Input: part model. Units: mm. Frame: model coordinates. Face numbers are marked on the shaded views. A direction names the side the tool comes from. Give positions to 0.01 mm unless a question says otherwise; leave off trailing zeros. One line per item, written item: value. Start each with the question number.
(1) Access query for the marked faces 1, 2 and 3. Directions: +Z, -Z, +X, -X, +Y, -Y. A direction counts if a zero-diameter tool reaches every point of the face in a straight line with its end or side. Return the directions, or none.
(2) Pull-direction query (X, two-part tool) for the marked faces 4, 5, 6 and 7; classes: released by +X, released by -X, zero draft, split by the parting line, or undercut.
(3) Ray query, line 1 along Z through (x, y) = (0, -22); line 2 along Y through (x, z) = (0, 8) (3 decimals); line 3 along Z through (x, y) = (0, 20.7). Return the intervals inside material, ascending. Write a range as from..to.
(4) Pin query (flat end, axial travel): P1, Ø1.5, axis at y = -1, z = -5, coming from the +X side; P2, Ø6, axis at y = 12.5, z = -14.5, coming from the -X side; P3, Ø6, axis at x = 18.5, z = 10, coming from the +Y side. Return the tip coordinate at first contact, or that it passes through.
```python
from build123d import *

# Parameters (mm, degrees)
SKETCH_2_W                       = 64.02174429
SKETCH_2_H                       = 9.248919907
CUT_EXTRUDE_1_DEPTH              = 49
HOLE_WIZARD_M4_2_D               = 3.3
HOLE_WIZARD_M4_2_DEPTH           = 5.5
HOLE_WIZARD_M4_2_TIP             = 0.991420021
HOLE_WIZARD_M6_2_D               = 5
HOLE_WIZARD_M6_2_DEPTH           = 5.5
HOLE_WIZARD_M6_2_TIP             = 1.502151548
HOLE_WIZARD_M4_3_D               = 3.3
HOLE_WIZARD_M4_3_DEPTH           = 10.1
HOLE_WIZARD_M4_3_TIP             = 0.991420021
HOLE_WIZARD_M4_3_ON_FACE_2_D     = 3.3
HOLE_WIZARD_M4_3_ON_FACE_2_DEPTH = 10.1
HOLE_WIZARD_M4_3_ON_FACE_2_TIP   = 0.991420021


with BuildPart() as part:
    # 草图1 → 旋转1 (revolve)
    with BuildSketch(Plane(origin=(0, 0, 0), x_dir=(1, 0, 0), z_dir=(0, 1, 0)), mode=Mode.PRIVATE) as revolve_1_sk:
        Polygon((25.4, 19), (25.4, -19), (17, -19), (17, -14.5), (17.6, -14.5), (17.6, -13.5), (15.875, -13.5), (15.875, -4), (16.975, -4), (16.975, 4), (15.875, 4), (15.875, 13.5), (17.6, 13.5), (17.6, 14.5), (17, 14.5), (17, 19), align=None)
    revolve(revolve_1_sk.sketch.rotate(Axis((0, 0, -31.9390681), (0, 0, 1)), 180), axis=Axis((0, 0, -31.9390681), (0, 0, 1)))  # turned: the seam where the file's is

    # 草图2 → 切除-拉伸1 (cut)
    with BuildSketch(Plane.XY.offset(19)):
        with Locations((-1.141100508, 29.124459954)):
            Rectangle(SKETCH_2_W, SKETCH_2_H)
        with Locations((-1.141100508, -29.124459954)):
            Rectangle(SKETCH_2_W, SKETCH_2_H)
    extrude(amount=-CUT_EXTRUDE_1_DEPTH, mode=Mode.SUBTRACT)

    # M4 螺纹孔2
    with Locations(Plane(origin=(0, 24.5, 0), x_dir=(1, 0, 0), z_dir=(0, 1, 0))):
        with Locations((0, 0)):
            Hole(HOLE_WIZARD_M4_2_D / 2, depth=HOLE_WIZARD_M4_2_DEPTH)
            with Locations((0, 0, -(HOLE_WIZARD_M4_2_DEPTH + HOLE_WIZARD_M4_2_TIP / 2))):  # 118° drill point
                Cone(0, HOLE_WIZARD_M4_2_D / 2, HOLE_WIZARD_M4_2_TIP, mode=Mode.SUBTRACT)

    # M6 螺纹孔2
    with Locations(Plane(origin=(0, -24.5, 0), x_dir=(-1, 0, 0), z_dir=(0, -1, 0))):
        with Locations((0, 0)):
            Hole(HOLE_WIZARD_M6_2_D / 2, depth=HOLE_WIZARD_M6_2_DEPTH)
            with Locations((0, 0, -(HOLE_WIZARD_M6_2_DEPTH + HOLE_WIZARD_M6_2_TIP / 2))):  # 118° drill point
                Cone(0, HOLE_WIZARD_M6_2_D / 2, HOLE_WIZARD_M6_2_TIP, mode=Mode.SUBTRACT)

    # M4 螺纹孔3
    with Locations(Plane(origin=(21.997045256, 12.7, 0), x_dir=(-0.5, 0.866025404, 0), z_dir=(0.866025404, 0.5, 0))):
        with Locations((0, 0)):
            Hole(HOLE_WIZARD_M4_3_D / 2, depth=HOLE_WIZARD_M4_3_DEPTH)
            with Locations((0, 0, -(HOLE_WIZARD_M4_3_DEPTH + HOLE_WIZARD_M4_3_TIP / 2))):  # 118° drill point
                Cone(0, HOLE_WIZARD_M4_3_D / 2, HOLE_WIZARD_M4_3_TIP, mode=Mode.SUBTRACT)

    # M4 螺纹孔3 on face 2
    with Locations(Plane(origin=(-21.997045256, 12.7, 0), x_dir=(-0.500000175, -0.866025303, 0), z_dir=(-0.866025303, 0.500000175, 0))):
        with Locations((0, 0)):
            Hole(HOLE_WIZARD_M4_3_ON_FACE_2_D / 2, depth=HOLE_WIZARD_M4_3_ON_FACE_2_DEPTH)
            with Locations((0, 0, -(HOLE_WIZARD_M4_3_ON_FACE_2_DEPTH + HOLE_WIZARD_M4_3_ON_FACE_2_TIP / 2))):  # 118° drill point
                Cone(0, HOLE_WIZARD_M4_3_ON_FACE_2_D / 2, HOLE_WIZARD_M4_3_ON_FACE_2_TIP, mode=Mode.SUBTRACT)


solid = part.part
```
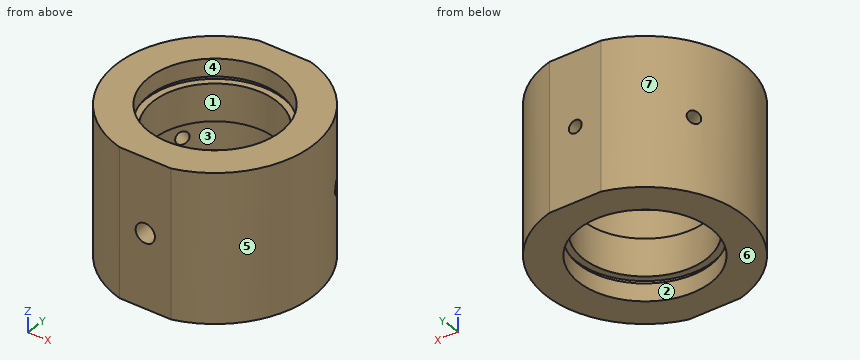
Output values:
1. face 1: +Z, -Z
1. face 2: -Z
1. face 3: none
2. face 4: undercut
2. face 5: released by +X
2. face 6: zero draft
2. face 7: released by -X
3. line 1: z = -19..-2.5, 2.5..19
3. line 2: y = -24.5..-15.875, 15.875..24.5
3. line 3: z = -19..-1.65, 1.65..19
4. P1: stops at x = 25.4
4. P2: stops at x = -23.56
4. P3: stops at y = 20.12
